Autodesk Inventor part; units mm, degrees
ref_plane "YZ Plane" through (0, 0, 0) normal (1, 0, 0) x (0, 1, 0)
ref_plane "XZ Plane" through (0, 0, 0) normal (0, 1, 0) x (-1, 0, 0)
ref_plane "XY Plane" through (0, 0, 0) normal (0, 0, 1) x (1, 0, 0)
sketch "Sketch1" plane through (0, 0, 0) normal (0, 0, 1) x (1, 0, 0)
  line L0 (9.525, 22.225) -> (9.525, -22.225)
  line L1 (9.525, -22.225) -> (-9.525, -22.225)
  line L2 (-9.525, -22.225) -> (-9.525, 22.225)
  line L3 (-9.525, 22.225) -> (9.525, 22.225)
  line L4 (12.7, 25.4) -> (-12.7, 25.4)
  line L5 (-12.7, 25.4) -> (-12.7, -25.4)
  line L6 (-12.7, -25.4) -> (12.7, -25.4)
  line L7 (12.7, -25.4) -> (12.7, 25.4)
  point P0 (0, 0)
  point P1 (0, 0)
extrude "Extrusion1" add sketch "Sketch1" along normal blind 393.7
sketch "Sketch2" plane through (12.7, -25.4, 0) normal (1, 0, 0) x (0, 0, -1)
  circle A0 centre (-196.85, 18.9017) radius 14.2875
  line L0 (-393.7, 0) -> (-393.7, 50.8)
  line L1 (0, 50.8) -> (0, 0)
  point P0 (0, 25.4)
  dimension "d2" = 28.575
  dimension "d22" = 196.85
extrude "Extrusion2" cut sketch "Sketch2" against normal blind 25.4
sketch "Sketch3" plane through (12.7, -25.4, 0) normal (1, 0, 0) x (0, 0, -1)
  circle A0 centre (-196.85, 18.9017) radius 14.2875
  circle A1 centre (-330.2, 25.4) radius 14.2875
  circle A2 centre (-63.5, 25.4) radius 14.2875
  line L0 (-393.7, 0) -> (-393.7, 50.8)
  line L1 (0, 0) -> (0, 50.8)
  point P0 (0, 25.4)
  dimension "d10" = 28.575
  dimension "d13" = 28.575
  dimension "d17" = 6.4983
  dimension "d20" = 63.5
  dimension "d21" = 63.5
extrude "Extrusion3" cut sketch "Sketch3" against normal blind 25.4 contours A1 | A2
properties part number "side 1"
Verification items for the finished model (mm, model axes). A direction names the side the tool comes from. Give positions to 0.01 mm unless a question says otherwise; leave off trailing zeros. Write each loop counter-clockwise with the first axis right and the second up, starting at its lowest first coordinate (ties: lowest second). Pieces come first, ordered by that corner, then holes. Notation, with made-up numbers: (-22.75, 76) -> (-12.75, 76) arc R31 cw to (-12.75, 113) -> close; hole circle Ø9 at (86.5, 0). An arc over 180 degrees is marked (long way). Use CSV: the item, a comma, the result in double quotes.
(1) Sectioned sample at C-C (z = 249). Record the cut outline in (x, y) (3 decimals), plus the area to 3 significant figures.
Derived:
outline,"(-12.7, -25.4) -> (12.7, -25.4) -> (12.7, 25.4) -> (-12.7, 25.4) -> close; hole (-9.525, -22.225) -> (9.525, -22.225) -> (9.525, 22.225) -> (-9.525, 22.225) -> close"
area,"444 mm^2"
(2) Sectioned sample at B-B (z = 330.2). Record the cut outline in (x, y) (1 decimal).
Derived:
outline,"(-12.7, -25.4) -> (12.7, -25.4) -> (12.7, -14.3) -> (9.5, -14.3) -> (9.5, -22.2) -> (-9.5, -22.2) -> (-9.5, -14.3) -> (-12.7, -14.3) -> close; (-12.7, 14.3) -> (-9.5, 14.3) -> (-9.5, 22.2) -> (9.5, 22.2) -> (9.5, 14.3) -> (12.7, 14.3) -> (12.7, 25.4) -> (-12.7, 25.4) -> close"
(3) Set-up check for faces 1 (the flat face through (0, 22.225, 194)), 2 (the cylindrical face through (-11.09, 0.628, 77.774)): record each of +Z, -Z, +X, -X, +Y, -Y from which the full face is reachable in a straight line by a thin tool's end or side.
Derived:
face 1,"+Z, -Z"
face 2,"+X, -X"
(4) Release check for a two-part mould opening along Z. For faces 3 (the flat face through (0, -22.225, 194)), 4 (the flat face through (-10, -2, 0)), 5 (the flat face through (-10, -2, 393.7)), 6 (the cylindrical face through (-11.09, -11.97, 183.65)) record: +Z half, -Z half, draft (parallel to the pull), parting line (faces both ways), or undercut.
Derived:
face 3,"draft"
face 4,"-Z half"
face 5,"+Z half"
face 6,"undercut"
(5) Sectioned sample at D-D (y = 0). Give the number of separate pieces and of enclosed holes in the cut face, plus the area to 3 significant figures.
Derived:
separate pieces,"8"
enclosed holes,"0"
area,"1,980 mm^2"
(6) Material ranges on L1, parallel to X at y = -9.5, z = 151.5 (3 decimals); L2, parallel to Y at x = -10.2, z = 330.2; L3, parallel to Y at x = -10.75, z = 196.85, recorded low to high.
Derived:
L1,"x = -12.7 to -9.525, 9.525 to 12.7"
L2,"y = -25.4 to -14.29, 14.29 to 25.4"
L3,"y = -25.4 to -20.79, 7.79 to 25.4"
(7) Sectioned sample at A-A (x = -3.5). Record the cut outline in (y, z) (3 decimals), plus the area to 3 significant figures.
Derived:
outline,"(-25.4, 0) -> (-22.225, 0) -> (-22.225, 393.7) -> (-25.4, 393.7) -> close; (22.225, 0) -> (25.4, 0) -> (25.4, 393.7) -> (22.225, 393.7) -> close"
area,"2,500 mm^2"
